Geometry check sheet. Reference: the model listing, model coordinates, mm. Coordinates: 2 decimals unless noted, no trailing zeros. Order: outer loops, then holes, each group sorted by start corner. A loop starts at its lowest first (then second) coordinate and runs counter-clockwise, first axis right, second up. Notation, with made-up numbers: (51.5, 49.25) - (92.5, 49.25) arc R25 cw to (92.5, 85.25) - close; hole circle Ø7 at (64.25, -12.5). An arc over 180 degrees is marked (long way). Return JSON: item names as keys, results as strings. Group by question number.
Item 1: Section check D-D on y = -18.5. Enter the section's corners in (x, z).
Item 2: Scan lines: probe 1 along Y at (x, z) = (-19, 1.75); probe 2 along Z at (x, y) = (56, -30); probe 3 along Y at (x, z) = (-88.5, -2.6). Record each from-to range of solid material in increasing order.
Item 3: Gauge pin test, flat ends, axial feed: pin 1 (2.5 mm diameter, centred on x = -15, z = -2, fed in from -Y); pin 2 (1.5 mm diameter, centred on y = -50, z = 1.5, fed in from -X); pin 3 (2.5 mm diameter, centred on x = -103, z = 1.5, fed in from -Y). Record the tip position at first contact, or that the pin passes through.
Item 4: Section check C-C on y = -108. Enter the section's corners in (x, z).
Item 5: Section check A-A on z = -1.3. Enter the section's corners in (x, y), then the cut area to 3 significant figures.
Item 6: Section check B-B on x = -15. Enter the section's corners in (y, z), then the cut area to 3 significant figures.
from build123d import *

# Parameters (mm, degrees)
F1_DEPTH = 3
F3_DEPTH = 3
F4_W     = 24
F4_H     = 3
F5_DEPTH = 3
F6_W     = 33.9326828589
F6_H     = 3
F7_DEPTH = 3


with BuildPart() as f1:
    # F0 (on Top) → F1 (new body)
    with BuildSketch(Plane.XY):
        with BuildLine():
            ThreePointArc((70.5214165197, -55.9710955009), (44.5935670538, -16.2265064733), (0, 0))
            Line((0, 0), (-115, 0))
            Line((-115, 0), (-115, -30))
            Line((-115, -30), (-75, -30))
            Line((-75, -30), (-33.1492031744, -54.1625688131))
            Line((-33.1492031744, -54.1625688131), (0, -54.1625688131))
            ThreePointArc((0, -54.1625688131), (24.3504571603, -62.4284352014), (38.6370330516, -83.809807009))
            Line((38.6370330516, -83.809807009), (57.1011837292, -152.7189554564))
            Line((57.1011837292, -152.7189554564), (95.7382167807, -142.3661936523))
            Line((95.7382167807, -142.3661936523), (70.5214165197, -55.9710955009))
        make_face()
    extrude(amount=-F1_DEPTH)

    # F2 (on face) → F3 (join)
    with BuildSketch(Plane.XY):
        with BuildLine():
            ThreePointArc((0, -51.1625688131), (26.1767414474, -60.0483751805), (41.5348105304, -83.0333498737))
            Line((41.5348105304, -83.0333498737), (59.2225040727, -149.0447208423))
            Line((59.2225040727, -149.0447208423), (91.9989588014, -140.262296267))
            Line((91.9989588014, -140.262296267), (67.629756974, -56.7711490177))
            ThreePointArc((67.629756974, -56.7711490177), (42.7604972061, -18.6017091288), (-0.0410552786, -3))
            Line((-0.0410552786, -3), (-112, -3))
            Line((-112, -3), (-112, -27))
            Line((-112, -27), (-74.1961524227, -27))
            Line((-74.1961524227, -27), (-32.3453555971, -51.1625688131))
            Line((-32.3453555971, -51.1625688131), (0, -51.1625688131))
        make_face()
    extrude(amount=F3_DEPTH)

    # F4 (on face) → F5 (join)
    with BuildSketch(Plane(origin=(-112, 0, 0), x_dir=(0, -1, 0), z_dir=(-1, 0, 0))):
        with Locations((15, 1.5)):
            Rectangle(F4_W, F4_H)
    extrude(amount=F5_DEPTH)

    # F6 (on face) → F7 (join)
    with BuildSketch(Plane(origin=(41.2283357456, -153.866243714, 0), x_dir=(0.9659258263, 0.2588190451, 0), z_dir=(0.2588190451, -0.9659258263, 0))):
        with Locations((35.5952752848, 1.5)):
            Rectangle(F6_W, F6_H)
    extrude(amount=F7_DEPTH)


solid = f1.part
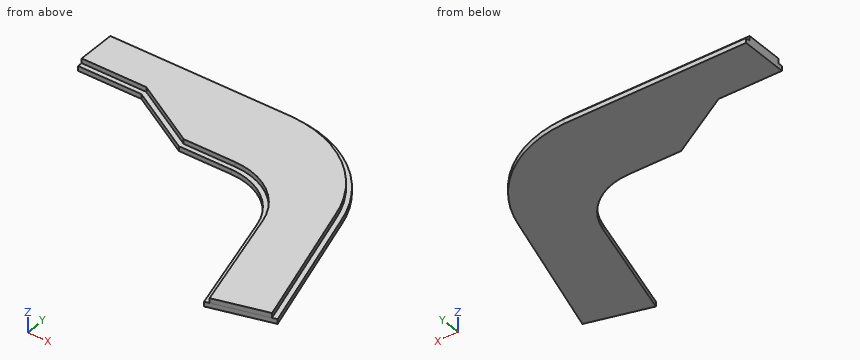
Computed:
{
 "1": {"outline": "(-115, -3) - (47.32, -3) - (47.32, 0) - (42.63, 0) - (42.63, 3) - (-115, 3) - close"},
 "2": {"probe 1": "y = -51.16 to -3", "probe 2": "z = -3 to 0", "probe 3": "y = -30 to 0"},
 "3": {"pin 1": "stops at y = -54.16", "pin 2": "stops at x = -35.66", "pin 3": "stops at y = -27"},
 "4": {"outline": "(45.12, -3) - (85.71, -3) - (85.71, 0) - (82.58, 0) - (82.58, 3) - (48.22, 3) - (48.22, 0) - (45.12, 0) - close"},
 "5": {"outline": "(-115, -30) - (-75, -30) - (-33.15, -54.16) - (0, -54.16) arc R40 cw to (38.64, -83.81) - (57.1, -152.72) - (95.74, -142.37) - (70.52, -55.97) arc R75 ccw to (0, 0) - (-115, 0) - close", "area": "11,500 mm²"},
 "6": {"outline": "(-54.16, -3) - (0, -3) - (0, 0) - (-3, 0) - (-3, 3) - (-51.16, 3) - (-51.16, 0) - (-54.16, 0) - close", "area": "307 mm²"}
}
